Input: part model. Units: mm. Frame: model coordinates. A direction names the side the tool comes from. Round coordinates to 2 decimals unless told otherwise and drop trailing zeros. Order: outer loops, then holes, each group sorted by start corner. A loop starts at its lowest first (then second) coordinate and runs counter-clockwise, first axis right, second up.
Item 1: Line query: L1, parallel to Y at x = 13.35, z = 0.6; L2, parallel to X at y = -18, z = 0.8; L3, parallel to Y at x = 14, z = 0.15. Output: solid intervals per line, ascending.
Item 2: First-contact query: pin 1 (0.6 mm diameter, centred on y = -19.5, z = 1, fed in from +X); pin 2 (0.6 mm diameter, centred on y = -19.5, z = 0.5, fed in from -X); pin 3 (1 mm diameter, centred on x = 8.5, z = 1.5, fed in from -Y). Flat tips, straight axial feed; report the tip coordinate or a pass-through.
Item 3: Cut plane D-D on x = 9. Output: boundary loops of the cut face in (y, z), then the cut area to 3 significant figures.
Item 4: Reachability of faces 1 (the flat face through (8.5, -19, 1)), 2 (the flat face through (0, -17.1, 1)), 3 (the flat face through (0, -22.2, 1)), 4 (the flat face through (-8.5, -20, 1)) from +Z, -Z, +X, -X, +Y, -Y: full face, straight path, thin tool, end or side. Return the list, or none.
Item 5: Mould query, pull axis X, two halves, no side actions, for faces 5 (the flat face through (0, -1, 0)), 6 (the flat face through (0, -14.2, 1)), 7 (the flat face through (-7, -12, 1)), 8 (the cylindrical face through (-8.215, -21.899, 1.014)). Classes: released by +X, released by -X, zero draft, split by the parting line, or undercut.
Item 6: Cut plane C-C on z = 1.15. Output: boundary loops of the cut face in (x, y), then the cut area to 3 significant figures.
Item 7: Cut plane A-A on x = 0. Output: boundary loops of the cut face in (y, z).
Item 8: Cut plane B-B on y = -6.1. Output: boundary loops of the cut face in (x, z).
Autodesk Inventor part; units mm, degrees
ref_plane "YZ Plane" through (0, 0, 0) normal (1, 0, 0) x (0, 1, 0)
ref_plane "XZ Plane" through (0, 0, 0) normal (0, 1, 0) x (-1, 0, 0)
ref_plane "XY Plane" through (0, 0, 0) normal (0, 0, 1) x (1, 0, 0)
sketch "Náčrt1" plane through (0, 0, 0) normal (0, 0, 1) x (1, 0, 0)
  arc A0 (8.5, -16.6565) -> (-8.5, -16.6565) centre (0, 0) ccw
  line L0 (8.5, -16.6565) -> (8.5, -22.2)
  line L1 (8.5, -22.2) -> (-8.5, -22.2)
  line L2 (-8.5, -22.2) -> (-8.5, -16.6565)
  line L3 (0, -18.7455) -> (8.5, -22.2) construction
  line L4 (0, -18.7455) -> (-8.5, -22.2) construction
  line L5 (0, 18.7) -> (0, -18.7455)
  line L6 (-13.35, 6.1) -> (13.35, 6.1)
  line L7 (13.35, 6.1) -> (13.35, -6.1)
  line L8 (13.35, -6.1) -> (-13.35, -6.1)
  line L9 (-13.35, -6.1) -> (-13.35, 6.1)
  line L10 (-13.35, 6.1) -> (13.35, -6.1) construction
  line L11 (13.35, 6.1) -> (-13.35, -6.1) construction
  circle A1 centre (-13.35, 6.1) radius 2.75
  circle A2 centre (-13.35, 6.1) radius 1.7
  circle A3 centre (-13.35, -6.1) radius 2.75
  circle A4 centre (-13.35, -6.1) radius 1.7
  circle A5 centre (13.35, -6.1) radius 2.75
  circle A6 centre (13.35, -6.1) radius 1.7
  circle A7 centre (13.35, 6.1) radius 2.75
  circle A8 centre (13.35, 6.1) radius 1.7
  line L12 (-7, -9.2) -> (7, -9.2)
  line L13 (7, -9.2) -> (7, -14.2)
  line L14 (7, -14.2) -> (-7, -14.2)
  line L15 (-7, -14.2) -> (-7, -9.2)
  line L16 (-7, -9.2) -> (7, -14.2) construction
  line L17 (7, -9.2) -> (-7, -14.2) construction
  line L18 (-3.55, -20.2) -> (3.55, -20.2)
  line L19 (3.55, -20.2) -> (3.55, -17.1)
  line L20 (3.55, -17.1) -> (-3.55, -17.1)
  line L21 (-3.55, -17.1) -> (-3.55, -20.2)
  line L22 (-3.55, -20.2) -> (3.55, -17.1) construction
  line L23 (3.55, -20.2) -> (-3.55, -17.1) construction
  point P0 (0, -11.7)
  point P1 (0, -18.65)
  point P2 (7, -6.1)
  point P3 (-7, -6.1)
  dimension "d0" = 37.4
  dimension "d1" = 17
  dimension "d2" = 22.2
  dimension "d3" = 26.7
  dimension "d4" = 12.2
  dimension "d5" = 5.5
  dimension "d6" = 3.4
  dimension "d7" = 5.5
  dimension "d8" = 3.4
  dimension "d9" = 5.5
  dimension "d10" = 3.4
  dimension "d11" = 5.5
  dimension "d12" = 3.4
  dimension "d15" = 14
  dimension "d16" = 5
  dimension "d21" = 7.1
  dimension "d22" = 3.1
  dimension "d23" = 2
  dimension "d24" = 8
extrude "Vysunutí1" add sketch "Náčrt1" along normal blind 2 contours L6 A7 L7 A5 L8 L5 | L5 L8 A3 L9 A1 L6 | L0 L1 L2 A0 | A1 L9 A2 L6 | L6 A2 L9 A1 | A7 L7 A8 L6 | L6 A8 L7 A7 | A5 L7 A6 L8 | L8 A6 L7 A5 | A3 L9 A4 L8 | L8 A4 L9 A3
fillet "Zaoblení1" radius 2 2 edges at (-8.5, -16.6565, 1) (8.5, -16.6565, 1)
fillet "Zaoblení2" radius 1 2 edges at (8.5, -22.2, 1) (-8.5, -22.2, 1)
fillet "Zaoblení3" radius 1 4 edges at (-7, -9.2, 1) (7, -9.2, 1) (-7, -14.2, 1) (7, -14.2, 1)
properties part number "Držák-Disp"
From the geometry:
1. L1: y = -13.09 to -7.8, -4.4 to 4.4, 7.8 to 13.09
1. L2: x = -8.5 to -3.55, 3.55 to 8.5
1. L3: y = -12.4 to -7.67, -4.53 to 4.53, 7.67 to 12.4
2. pin 1: stops at x = 8.5
2. pin 2: stops at x = -8.5
2. pin 3: stops at y = -22.07
3. outline: (-16.52, 0) - (16.39, 0) - (16.39, 2) - (-16.52, 2) - close
3. area: 65.8 mm2
4. face 1: +Z, -Z, +X, -Y
4. face 2: +Z, -Z
4. face 3: +Z, -Z, +X, -X, -Y
4. face 4: +Z, -Z, -X, -Y
5. face 5: zero draft
5. face 6: undercut
5. face 7: undercut
5. face 8: released by -X
6. outline: (-9.49, -16.12) arc R2 cw to (-8.5, -17.84) - (-8.5, -21.2) arc R1 ccw to (-7.5, -22.2) - (7.5, -22.2) arc R1 ccw to (8.5, -21.2) - (8.5, -17.84) arc R2 cw to (9.49, -16.12) arc R18.7 ccw (long way) to start; hole circle Ø3.4 at (-13.35, -6.1); hole circle Ø3.4 at (-13.35, 6.1); hole (-7, -13.2) arc R1 ccw to (-6, -14.2) - (6, -14.2) arc R1 ccw to (7, -13.2) - (7, -10.2) arc R1 ccw to (6, -9.2) - (-6, -9.2) arc R1 ccw to (-7, -10.2) - close; hole (-3.55, -20.2) - (3.55, -20.2) - (3.55, -17.1) - (-3.55, -17.1) - close; hole circle Ø3.4 at (13.35, -6.1); hole circle Ø3.4 at (13.35, 6.1)
6. area: 1,040 mm2
7. outline: (-22.2, 0) - (-20.2, 0) - (-20.2, 2) - (-22.2, 2) - close; (-17.1, 0) - (-14.2, 0) - (-14.2, 2) - (-17.1, 2) - close; (-9.2, 0) - (18.7, 0) - (18.7, 2) - (-9.2, 2) - close
8. outline: (-17.68, 0) - (-15.05, 0) - (-15.05, 2) - (-17.68, 2) - close; (-11.65, 0) - (11.65, 0) - (11.65, 2) - (-11.65, 2) - close; (15.05, 0) - (17.68, 0) - (17.68, 2) - (15.05, 2) - close
